```python
from build123d import *

# Parameters (mm, degrees)
EXTRUDE1_DEPTH = 25.4


with BuildPart() as part:
    # Sketch1 → Extrude1 (new body)
    with BuildSketch(Plane(origin=(0, 0, 0), x_dir=(1, 0, 0), z_dir=(0, 1, 0))):
        with BuildLine():
            Line((-17.4625, 0), (17.4625, 0))
            ThreePointArc((17.4625, 0), (18.585032015, 0.464967985), (19.05, 1.5875))
            Line((19.05, 1.5875), (19.05, 76.234673011))
            ThreePointArc((19.05, 76.234673011), (18.965751581, 76.744958163), (18.721948428, 77.20108178))
            Line((18.721948428, 77.20108178), (1.259448428, 99.958654853))
            ThreePointArc((1.259448428, 99.958654853), (0, 100.579746085), (-1.259448428, 99.958654853))
            Line((-1.259448428, 99.958654853), (-18.721948428, 77.20108178))
            ThreePointArc((-18.721948428, 77.20108178), (-18.965751581, 76.744958163), (-19.05, 76.234673011))
            Line((-19.05, 76.234673011), (-19.05, 1.5875))
            ThreePointArc((-19.05, 1.5875), (-18.585032015, 0.464967985), (-17.4625, 0))
        make_face()
    extrude(amount=EXTRUDE1_DEPTH)


solid = part.part
```
Geometry: final body of the model. Coordinates: model frame, mm. Give positions to 0.01 mm unless a question says otherwise; leave off trailing zeros. Order: outer loops, then holes, each group sorted by start corner. A loop starts at its lowest first (then second) coordinate and runs counter-clockwise, first axis right, second up. Notation, with made-up numbers: (32, -16.5) -> (68, -16.5) arc R15 ccw to (68, -11.5) -> close; hole circle Ø8 at (83.25, 24.5). An arc over 180 degrees is marked (long way). Write each question's results on one line, items separated by ' | '. Start each with the question number.
1) First-contact query: pin 1 (1 mm diameter, centred on x = 7.5, y = 5.5, fed in from -Z); pin 2 (1.5 mm diameter, centred on x = 6, y = 3.5, fed in from -Z); pin 3 (5 mm diameter, centred on x = 11, y = 11, fed in from -Z). Flat tips, straight axial feed; report the tip coordinate or a pass-through.
2) Section B-B (x = 8.5). Return loops of the section in (y, z).
3) Line query: line 1 (Z direction, x = 8, y = 4.25); line 2 (Z direction, x = 9.5, y = 14.25); line 3 (X direction, y = 3.25, z = -88). Output: solid intervals per line, ascending. Write a range as from..to.
4) Section C-C (z = -86). Return loops of the section in (x, y).
Calculated:
1) pin 1: z = -92.48 | pin 2: z = -94.76 | pin 3: z = -90.52
2) outline: (0, -90.52) -> (25.4, -90.52) -> (25.4, 0) -> (0, 0) -> close
3) line 1: -91.17..0 | line 2: -89.22..0 | line 3: -10.44..10.44
4) outline: (-11.97, 0) -> (11.97, 0) -> (11.97, 25.4) -> (-11.97, 25.4) -> close
